The listing builds one solid part. Answer for the finished solid, in the listing's coordinates (mm). Face numbers are marked on the shaded views. A direction names the side the tool comes from. Round coordinates to 2 decimals unless told otherwise and drop trailing zeros. Loops run counter-clockwise (first coordinate to the right, second up) from the corner with the lowest first, then second, coordinate; pieces in that order, holes last. Notation, with made-up numbers: (-3, 73.5) -> (53, 73.5) arc R10 ccw to (53, 80.5) -> close; hole circle Ø10 at (22.25, 82). An arc over 180 degrees is marked (long way). Answer in a Markdown table with one row per item. Add a question column.
Autodesk Inventor part; units mm, degrees
ref_plane "Work Plane1" through (-77, -15, -14.9044) normal (0, 0, 1) x (1, 0, 0)
ref_plane "YZ Plane" through (0, 0, 0) normal (1, 0, 0) x (0, 1, 0)
ref_plane "XZ Plane" through (0, 0, 0) normal (0, 1, 0) x (-1, 0, 0)
sketch "Sketch1" plane through (0, 0, 0) normal (0, 0, 1) x (1, 0, 0)
  circle A0 centre (-100.25, -3.5) radius 1.5
  circle A1 centre (-100.25, -11.5) radius 1.5
  line L0 (-104, 0) -> (-96.5, 0)
  line L1 (-104, 0) -> (-104, -15)
  line L2 (-96.5, -15) -> (-104, -15)
  line L3 (-96.5, 0) -> (-96.5, -15)
  circle A2 centre (-85.75, -3.5) radius 1.5
  circle A3 centre (-85.75, -11.5) radius 1.5
  line L4 (-90.5, 0) -> (-81, 0)
  line L5 (-90.5, 0) -> (-90.5, -15)
  line L6 (-81, -15) -> (-90.5, -15)
  line L7 (-81, 0) -> (-81, -15)
  circle A4 centre (-15.25, -11.5) radius 1.5
  circle A5 centre (-15.25, -3.5) radius 1.5
  line L8 (-20, 0) -> (-10.5, 0)
  line L9 (-20, 0) -> (-20, -15)
  line L10 (-10.5, -15) -> (-20, -15)
  line L11 (-10.5, 0) -> (-10.5, -15)
  circle A6 centre (-0.75, -3.5) radius 1.5
  circle A7 centre (-0.75, -11.5) radius 1.5
  line L12 (-4.5, 0) -> (3, 0)
  line L13 (-4.5, 0) -> (-4.5, -15)
  line L14 (3, -15) -> (-4.5, -15)
  line L15 (3, 0) -> (3, -15)
  line L16 (-104, -15) -> (3, -15)
  line L17 (3, -15) -> (3, 0)
  line L18 (3, 0) -> (-104, 0)
  line L19 (-104, 0) -> (-104, -15)
  line L20 (-50.5, -15) -> (-50.5, 0)
  line L21 (-70.5, -11.5) -> (-70.5, -3.5)
  line L22 (-70.5, -3.5) -> (-30.5, -3.5)
  line L23 (-30.5, -3.5) -> (-30.5, -11.5)
  line L24 (-30.5, -11.5) -> (-70.5, -11.5)
  line L25 (-70.5, -11.5) -> (-30.5, -3.5) construction
  line L26 (-70.5, -3.5) -> (-30.5, -11.5) construction
  line L27 (-70.5, -3.5) -> (-81, 0)
  line L28 (-30.5, -3.5) -> (-20, 0)
  line L29 (-30.5, -11.5) -> (-20, -15)
  line L30 (-70.5, -11.5) -> (-81, -15)
  point P0 (0, 0)
  point P1 (-50.5, -7.5)
  dimension "d0" = 8
  dimension "d1" = 40
extrude "Extrusion1" add sketch "Sketch1" along normal blind 5 contours L0 L3 L2 L1 | L18 L5 L16 L3 | L4 L7 L6 L5 | L27 L21 L30 L7 | L22 L20 L24 L21 | L8 L11 L10 L9 | L9 L29 L23 L28 | L22 L23 L24 L20 | L18 L13 L16 L11 | L12 L15 L14 L13
sketch "Sketch2" plane through (0, 0, 5) normal (0, 0, 1) x (1, 0, 0)
  line L0 (-81, 0) -> (-104, 0)
  line L1 (-104, 0) -> (-104, -15)
  line L2 (-104, -15) -> (-81, -15)
  line L3 (-81, -15) -> (-70.5, -11.5)
  line L4 (-70.5, -11.5) -> (-30.5, -11.5)
  line L5 (-30.5, -11.5) -> (-20, -15)
  line L6 (-20, -15) -> (3, -15)
  line L7 (3, -15) -> (3, 0)
  line L8 (3, 0) -> (-20, 0)
  line L9 (-20, 0) -> (-30.5, -3.5)
  line L10 (-30.5, -3.5) -> (-70.5, -3.5)
  line L11 (-70.5, -3.5) -> (-81, 0)
  circle A0 centre (-100.25, -3.5) radius 1.5
  circle A1 centre (-100.25, -11.5) radius 1.5
  circle A2 centre (-85.75, -3.5) radius 1.5
  circle A3 centre (-85.75, -11.5) radius 1.5
  circle A4 centre (-15.25, -11.5) radius 1.5
  circle A5 centre (-15.25, -3.5) radius 1.5
  circle A6 centre (-0.75, -3.5) radius 1.5
  circle A7 centre (-0.75, -11.5) radius 1.5
  line L12 (-70.5, -11.5) -> (-30.5, -11.5)
  line L13 (-50.5, -11.5) -> (-50.5, -3.5)
  line L14 (-30.5, -3.5) -> (-70.5, -3.5)
  line L15 (-50.5, -7.5) -> (-60.5, -7.5)
  line L16 (-60.5, -7.5) -> (-70.5, -7.5)
  line L17 (-50.5, -7.5) -> (-40.5, -7.5)
  line L18 (-40.5, -7.5) -> (-30.5, -7.5)
  circle A8 centre (-70.5, -7.5) radius 1.5
  circle A9 centre (-60.5, -7.5) radius 1.5
  circle A10 centre (-50.5, -7.5) radius 1.5
  circle A11 centre (-40.5, -7.5) radius 1.5
  circle A12 centre (-30.5, -7.5) radius 1.5
  point P0 (0, 0)
  dimension "d4" = 10
  dimension "d5" = 10
  dimension "d6" = 10
  dimension "d7" = 10
  dimension "d8" = 3
  dimension "d9" = 3
  dimension "d10" = 3
  dimension "d11" = 3
  dimension "d12" = 3
extrude "Extrusion2" cut sketch "Sketch2" against normal blind 5 contours A8 | A9 L16 L15 | L15 L16 A9 | A12 | A11 L18 L17 | L17 L18 A11 | A10 L17 L13 | L13 L15 A10 | L17 A10 L13 | L13 A10 L15
fillet "Fillet1" radius 2 4 edges at (-104, 0, 2.5) (-104, -15, 2.5) (3, -15, 2.5) (3, 0, 2.5)
sketch "Sketch3" plane through (0, 0, 5) normal (0, 0, 1) x (1, 0, 0)
  arc A0 (3, -2) -> (1, 0) centre (1, -2) ccw
  line L0 (1, 0) -> (-20, 0)
  line L1 (-20, 0) -> (-30.5, -3.5)
  line L2 (-30.5, -3.5) -> (-70.5, -3.5)
  line L3 (-70.5, -3.5) -> (-81, 0)
  line L4 (-81, 0) -> (-102, 0)
  arc A1 (-102, 0) -> (-104, -2) centre (-102, -2) ccw
  line L5 (-104, -2) -> (-104, -13)
  arc A2 (-104, -13) -> (-102, -15) centre (-102, -13) ccw
  line L6 (-102, -15) -> (-81, -15)
  line L7 (-81, -15) -> (-70.5, -11.5)
  line L8 (-70.5, -11.5) -> (-30.5, -11.5)
  line L9 (-30.5, -11.5) -> (-20, -15)
  line L10 (-20, -15) -> (1, -15)
  arc A3 (1, -15) -> (3, -13) centre (1, -13) ccw
  line L11 (3, -13) -> (3, -2)
  circle A4 centre (-50.5, -7.5) radius 1.5
  circle A5 centre (-40.5, -7.5) radius 1.5
  circle A6 centre (-60.5, -7.5) radius 1.5
  circle A7 centre (-30.5, -7.5) radius 1.5
  circle A8 centre (-70.5, -7.5) radius 1.5
  circle A9 centre (-100.25, -3.5) radius 1.5
  circle A10 centre (-100.25, -11.5) radius 1.5
  circle A11 centre (-85.75, -3.5) radius 1.5
  circle A12 centre (-85.75, -11.5) radius 1.5
  circle A13 centre (-15.25, -11.5) radius 1.5
  circle A14 centre (-15.25, -3.5) radius 1.5
  circle A15 centre (-0.75, -3.5) radius 1.5
  circle A16 centre (-0.75, -11.5) radius 1.5
  line L12 (-55.5, -11.5) -> (-55.5, -3.5)
  line L13 (-55.5, -3.5) -> (-45.5, -3.5)
  line L14 (-45.5, -3.5) -> (-45.5, -11.5)
  line L15 (-45.5, -11.5) -> (-55.5, -11.5)
  circle A17 centre (-50.5, -7.5) radius 1.5
  line L16 (-55.5, -11.5) -> (-45.5, -3.5) construction
  line L17 (-55.5, -3.5) -> (-45.5, -11.5) construction
  point P0 (0, 0)
  dimension "d16" = 8
  dimension "d17" = 10
ref_plane "Work Plane1" through (-77, -15, -14.9044) normal (0, 0, 1) x (1, 0, 0)
extrude "Extrusion3" add sketch "Sketch3" against normal up to surface (19.9044 mm away) contours L14 L8 L12 L2
chamfer "Chamfer1" distance 2.5 angle 45 4 edges at (-45.5, -3.5, -7.4522) (-55.5, -3.5, -7.4522) (-45.5, -11.5, -7.4522) (-55.5, -11.5, -7.4522)
fillet "Fillet2" radius 3 6 edges at (-54.25, -10.25, 0) (-55.5, -7.5, 0) (-54.25, -4.75, 0) (-46.75, -10.25, 0) (-45.5, -7.5, 0) (-46.75, -4.75, 0)
fillet "Fillet3" radius 1 1 edges at (-50.5, -3.5, -14.9044)
fillet "Fillet4" radius 20 4 edges at (-70.5, -3.5, 2.5) (-30.5, -3.5, 2.5) (-70.5, -11.5, 2.5) (-30.5, -11.5, 2.5)
sketch "Sketch4" plane through (0, 0, 5) normal (0, 0, 1) x (1, 0, 0)
  circle A0 centre (-0.75, -11.5) radius 1.5
  circle A1 centre (-0.75, -3.5) radius 1.5
  circle A2 centre (-15.25, -3.5) radius 1.5
  circle A3 centre (-15.25, -11.5) radius 1.5
  circle A4 centre (-30.5, -7.5) radius 1.5
  circle A5 centre (-40.5, -7.5) radius 1.5
  circle A6 centre (-50.5, -7.5) radius 1.5
  line L0 (-33.7456, -3.5) -> (-67.2544, -3.5)
  arc A7 (-73.579, -2.4737) -> (-67.2544, -3.5) centre (-67.2544, 16.5) ccw
  line L1 (-73.579, -2.4737) -> (-81, 0)
  line L2 (-81, 0) -> (-102, 0)
  arc A8 (-102, 0) -> (-104, -2) centre (-102, -2) ccw
  line L3 (-104, -2) -> (-104, -13)
  arc A9 (-104, -13) -> (-102, -15) centre (-102, -13) ccw
  line L4 (-102, -15) -> (-81, -15)
  line L5 (-81, -15) -> (-73.579, -12.5263)
  arc A10 (-67.2544, -11.5) -> (-73.579, -12.5263) centre (-67.2544, -31.5) ccw
  line L6 (-67.2544, -11.5) -> (-33.7456, -11.5)
  arc A11 (-27.421, -12.5263) -> (-33.7456, -11.5) centre (-33.7456, -31.5) ccw
  line L7 (-27.421, -12.5263) -> (-20, -15)
  line L8 (-20, -15) -> (1, -15)
  arc A12 (1, -15) -> (3, -13) centre (1, -13) ccw
  line L9 (3, -13) -> (3, -2)
  arc A13 (3, -2) -> (1, 0) centre (1, -2) ccw
  line L10 (1, 0) -> (-20, 0)
  line L11 (-20, 0) -> (-27.421, -2.4737)
  arc A14 (-33.7456, -3.5) -> (-27.421, -2.4737) centre (-33.7456, 16.5) ccw
  circle A15 centre (-60.5, -7.5) radius 1.5
  circle A16 centre (-70.5, -7.5) radius 1.5
  circle A17 centre (-100.25, -3.5) radius 1.5
  circle A18 centre (-100.25, -11.5) radius 1.5
  circle A19 centre (-85.75, -3.5) radius 1.5
  circle A20 centre (-85.75, -11.5) radius 1.5
  line L12 (-100.25, -3.5) -> (-85.75, -11.5)
  circle A21 centre (-85.75, -3.5) radius 1.5
  line L13 (-85.75, -11.5) -> (-85.75, -3.5)
  circle A22 centre (-100.25, -11.5) radius 1.5
  line L14 (-85.75, -3.5) -> (-100.25, -11.5)
  circle A23 centre (-15.25, -11.5) radius 1.5
  line L15 (-0.75, -3.5) -> (-15.25, -11.5)
  line L16 (-15.25, -11.5) -> (-15.25, -3.5)
  circle A24 centre (-0.75, -11.5) radius 1.5
  line L17 (-15.25, -3.5) -> (-0.75, -11.5)
  circle A25 centre (-93, -7.5) radius 3
  circle A26 centre (-8, -7.5) radius 3
  point P0 (0, 0)
  dimension "d26" = 6
  dimension "d27" = 6
extrude "Extrusion4" cut sketch "Sketch4" against normal blind 5 contours A26 L15 L17 | L17 L15 A26 | L17 A26 L15 | L15 A26 L17 | A25 L14 L12 | L12 L14 A25 | L14 A25 L12 | L12 A25 L14
properties part number "carbon_fiber_fixer_1"
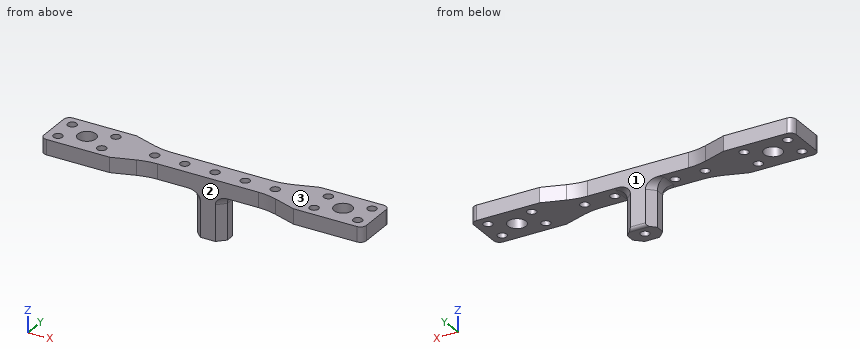
Item 1: Section C-C, the plane z = -12.5 is taken. Write down the section's boundary in (x, y).
Item 2: Section B-B, the plane x = -8 is taken. Write down the section's boundary in (y, z), and give its area (3 significant figures).
Item 3: Section D-D, the plane x = -60.5 is taken. Write down the section's boundary in (y, z).
Item 4: Flat-ended cylindrical pins translate along their axes: P1, Ø3.5, axis at x = -60.5, y = -7.5, coming from the +Z side; P2, Ø4, axis at x = -70.5, y = -7.5, coming from the -Z side; P3, Ø2.5, axis at y = -7, z = -12, coming from the -X side; P4, Ø2, axis at y = -11, z = -10.5, coming from the -X side. Find the tip coordinate at first contact, or state that the pin passes through.
Item 5: For the marked faces 1, 2 and 3, determine the directions among +Z, -Z, +X, -X, +Y, -Y from which every point of the face is accessible in a straight line to the end or side of a thin tool.
Item 6: Section A-A, the plane x = -100.25 is taken. Write down the section's boundary in (y, z).
Item 7: Consider L1, parallel to Y at x = -85.75, z = 2.7; L2, parallel to Y at x = -93, z = 3.5; L3, parallel to Z at x = -89, y = -8. Determine where each line is inside the solid, lowest interval first. Write a range as from..to.
Here are the results:
| question | item | result |
|---|---|---|
| 1 | outline | (-55.5, -9) -> (-53, -11.5) -> (-48, -11.5) -> (-45.5, -9) -> (-45.5, -6) -> (-48, -3.5) -> (-53, -3.5) -> (-55.5, -6) -> close; hole circle Ø3 at (-50.5, -7.5) |
| 2 | outline | (-15, 0) -> (-10.5, 0) -> (-10.5, 5) -> (-15, 5) -> close; (-4.5, 0) -> (0, 0) -> (0, 5) -> (-4.5, 5) -> close |
| 2 | area | 45.0 mm² |
| 3 | outline | (-11.5, 0) -> (-9, 0) -> (-9, 5) -> (-11.5, 5) -> close; (-6, 0) -> (-3.5, 0) -> (-3.5, 5) -> (-6, 5) -> close |
| 4 | P1 | stops at z = 5 |
| 4 | P2 | stops at z = 0 |
| 4 | P3 | stops at x = -55.5 |
| 4 | P4 | stops at x = -54.5 |
| 5 | face 1 | +Z, -Z, +Y |
| 5 | face 2 | +Z, -Z, -Y |
| 5 | face 3 | +Z, +X, -X, +Y, -Y |
| 6 | outline | (-15, 0) -> (-13, 0) -> (-13, 5) -> (-15, 5) -> close; (-10, 0) -> (-5, 0) -> (-5, 5) -> (-10, 5) -> close; (-2, 0) -> (0, 0) -> (0, 5) -> (-2, 5) -> close |
| 7 | L1 | y = -15..-13, -10..-5, -2..0 |
| 7 | L2 | y = -15..-10.5, -4.5..0 |
| 7 | L3 | z = 0..5 |
